from build123d import *

# Parameters (mm, degrees)
CYLINDER010_R     = 2.1
CYLINDER010_DEPTH = 30
CYLINDER011_R     = 2.1
CYLINDER011_DEPTH = 30
SKETCH002_R       = 1.8
SKETCH002_R_2     = 2.1
EXTRUDE001_DEPTH  = 5
BOX010_W          = 7
BOX010_H          = 3.6
BOX010_DEPTH      = 16
FILLET006_R       = 1.5
BOX009_W          = 7
BOX009_H          = 10
BOX009_DEPTH      = 24
FILLET005_R       = 3
SKETCH006_R       = 3
EXTRUDE005_DEPTH  = 9


with BuildPart() as insert_hole:
    # Cylinder010 → Cylinder010 (new body)
    with BuildSketch(Plane(origin=(7.6, 44.5, 0), x_dir=(1, 0, 0), z_dir=(0, 0, 1))):
        Circle(CYLINDER010_R)
    extrude(amount=CYLINDER010_DEPTH)


with BuildPart() as insert_hole_fusion:
    # Cylinder011 → Cylinder011 (new body)
    with BuildSketch(Plane(origin=(9.8, -45.6, 0), x_dir=(1, 0, 0), z_dir=(0, 0, 1))):
        Circle(CYLINDER011_R)
    extrude(amount=CYLINDER011_DEPTH)

    # Fusion010: union insert hole
    add(insert_hole.part)


with BuildPart() as pair_connector_extrude:
    # Sketch002 → Extrude001 (new body)
    with BuildSketch(Plane.XY):
        with BuildLine():
            Line((-36, -49), (0, -49))
            Line((0, -49), (36, -49))
            ThreePointArc((36, -49), (42.363961, -46.363961), (45, -40))
            Line((45, -40), (45, 0))
            Line((45, 0), (45, 40))
            ThreePointArc((45, 40), (42.363961, 46.363961), (36, 49))
            Line((36, 49), (0, 49))
            Line((0, 49), (-36, 49))
            ThreePointArc((-36, 49), (-42.363961, 46.363961), (-45, 40))
            Line((-45, 40), (-45, 0))
            Line((-45, 0), (-45, -40))
            ThreePointArc((-45, -40), (-42.363961, -46.363961), (-36, -49))
        make_face()
        with Locations((-18, 45)):
            Circle(SKETCH002_R, mode=Mode.SUBTRACT)
        with Locations((18, 45)):
            Circle(SKETCH002_R, mode=Mode.SUBTRACT)
        with Locations((-18, -45)):
            Circle(SKETCH002_R, mode=Mode.SUBTRACT)
        with Locations((18, -45)):
            Circle(SKETCH002_R, mode=Mode.SUBTRACT)
        with Locations((-41, 10)):
            Circle(SKETCH002_R_2, mode=Mode.SUBTRACT)
        with Locations((-41, -10)):
            Circle(SKETCH002_R_2, mode=Mode.SUBTRACT)
        with Locations((41, -10)):
            Circle(SKETCH002_R_2, mode=Mode.SUBTRACT)
        with Locations((41, 10)):
            Circle(SKETCH002_R_2, mode=Mode.SUBTRACT)
        with BuildLine():
            Line((-30, -42), (0, -42))
            Line((0, -42), (30, -42))
            ThreePointArc((30, -42), (34.949747, -39.949747), (37, -35))
            Line((37, -35), (37, 0))
            Line((37, 0), (37, 35))
            ThreePointArc((37, 35), (34.949747, 39.949747), (30, 42))
            Line((30, 42), (0, 42))
            Line((0, 42), (-30, 42))
            ThreePointArc((-30, 42), (-34.949747, 39.949747), (-37, 35))
            Line((-37, 35), (-37, 0))
            Line((-37, 0), (-37, -35))
            ThreePointArc((-37, -35), (-34.949747, -39.949747), (-30, -42))
        make_face(mode=Mode.SUBTRACT)
    extrude(amount=EXTRUDE001_DEPTH)


with BuildPart() as pair_connector_extrude_1:
    # Extrude001 placement: moved
    add(pair_connector_extrude.part.moved(Location((0, 0, 6.2))))


with BuildPart() as stand_hole_fillet:
    # Box010 → Box010 (new body)
    with BuildSketch(Plane(origin=(0, -1.8, 4), x_dir=(1, 0, 0), z_dir=(0, 0, 1))):
        with Locations((3.5, 1.8)):
            Rectangle(BOX010_W, BOX010_H)
    extrude(amount=BOX010_DEPTH)

    # Fillet006
    fillet006_edges = [stand_hole_fillet.edges().sort_by_distance(p)[0] for p in [
        (3.5, -1.8, 4),
        (3.5, -1.8, 20),
        (3.5, 1.8, 4),
        (3.5, 1.8, 20),
    ]]
    fillet(fillet006_edges, radius=FILLET006_R)


with BuildPart() as stand_hole_cut:
    # Box009 → Box009 (new body)
    with BuildSketch(Plane(origin=(0, -5, 0), x_dir=(1, 0, 0), z_dir=(0, 0, 1))):
        with Locations((3.5, 5)):
            Rectangle(BOX009_W, BOX009_H)
    extrude(amount=BOX009_DEPTH)

    # Fillet005
    fillet005_edges = [stand_hole_cut.edges().sort_by_distance(p)[0] for p in [
        (3.5, -5, 24),
        (3.5, 5, 24),
    ]]
    fillet(fillet005_edges, radius=FILLET005_R)

    # Cut005: cut stand hole fillet
    add(stand_hole_fillet.part, mode=Mode.SUBTRACT)


with BuildPart() as negative_stand_compound:
    # Compound022 base: copy of stand hole cut
    add(stand_hole_cut.part)


with BuildPart() as negative_stand_compound_1:
    # Compound022 placement: moved
    add(negative_stand_compound.part.moved(Location((-15.1, -45.9, 15.2))))


with BuildPart() as positive_stand_compound:
    # Compound023 base: copy of stand hole cut
    add(stand_hole_cut.part)


with BuildPart() as positive_stand_compound_1:
    # Compound023 placement: moved
    add(positive_stand_compound.part.moved(Location((-8.7, 46, 15.2))))


with BuildPart() as pair_connector_fusion_cut:
    # Sketch006 → Extrude005 (new body)
    with BuildSketch(Plane.XY):
        with BuildLine():
            Line((-22.841771, 51), (23.601032, 51))
            ThreePointArc((25.015246, 49.585786), (24.601032, 50.585786), (23.601032, 51))
            Line((25.015246, 49.585786), (25.015246, 42.214214))
            ThreePointArc((23.801032, 41), (24.659611, 41.355635), (25.015246, 42.214214))
            Line((23.801032, 41), (-23.041771, 41))
            ThreePointArc((-24.255985, 42.214214), (-23.90035, 41.355635), (-23.041771, 41))
            Line((-24.255985, 42.214214), (-24.255985, 49.585786))
            ThreePointArc((-22.841771, 51), (-23.841771, 50.585786), (-24.255985, 49.585786))
        make_face()
        with Locations((18, 45)):
            Circle(SKETCH006_R, mode=Mode.SUBTRACT)
        with Locations((-18, 45)):
            Circle(SKETCH006_R, mode=Mode.SUBTRACT)
        with BuildLine():
            Line((-22.399903, -41), (21.849301, -41))
            ThreePointArc((23.263515, -42.414214), (22.849301, -41.414214), (21.849301, -41))
            Line((23.263515, -42.414214), (23.263515, -49.785786))
            ThreePointArc((22.049301, -51), (22.90788, -50.644365), (23.263515, -49.785786))
            Line((22.049301, -51), (-22.599903, -51))
            ThreePointArc((-23.814117, -49.785786), (-23.458482, -50.644365), (-22.599903, -51))
            Line((-23.814117, -49.785786), (-23.814117, -42.414214))
            ThreePointArc((-22.399903, -41), (-23.399903, -41.414214), (-23.814117, -42.414214))
        make_face()
        with Locations((-18, -45)):
            Circle(SKETCH006_R, mode=Mode.SUBTRACT)
        with Locations((18, -45)):
            Circle(SKETCH006_R, mode=Mode.SUBTRACT)
    extrude(amount=EXTRUDE005_DEPTH)


with BuildPart() as pair_connector_fusion_cut_1:
    # Extrude005 placement: moved
    add(pair_connector_fusion_cut.part.moved(Location((0, 0, 6.2))))

    # Fusion008: union pair connector extrude, negative stand compound, positive stand compound
    add(pair_connector_extrude_1.part)
    add(negative_stand_compound_1.part)
    add(positive_stand_compound_1.part)

    # Cut007: cut insert hole fusion
    add(insert_hole_fusion.part, mode=Mode.SUBTRACT)


solid = pair_connector_fusion_cut_1.part
Read the model definition and answer for the solid it produces. Units are mm, in the model's axes. A direction names the side the tool comes from. Round coordinates to 2 decimals unless told otherwise and drop trailing zeros. Write each loop counter-clockwise with the first axis right and the second up, starting at its lowest first coordinate (ties: lowest second). Pieces come first, ordered by that corner, then holes.
1. Given pin 1 Ø3 at (y, z) = (-48, 33) entering from -X; pin 2 Ø3.5 at (x, y) = (41, -10) entering from +Z; pin 3 Ø10.5 at (x, y) = (-35.5, -5.5) entering from +Z; pin 4 Ø7.5 at (x, z) = (-12.5, 26) entering from -Y, each flat-ended and moving along its own axis, determine where each tip first touches the part or whether it passes through.
2. The part is cut by section C-C, the plane y = -30. Determine the outline of the cut face in (x, z).
3. Straight lines are drawn through the part: L1, parallel to Y at x = 18, z = 14; L2, parallel to X at y = 44.5, z = 10.5; L3, parallel to Y at x = -18, z = 7.6. For each, find the intervals that lie inside material, in ascending order.
4. The part is cut by section D-D, the plane y = 10. Determine the outline of the cut face in (x, z).
5. The part is cut by section A-A, the plane z = 27. Determine the outline of the cut face in (x, y), then the cut area to 3 significant figures.
6. The part is cut by section B-B, the plane x = -18. Determine the outline of the cut face in (y, z).
7. Determine the mould class of faces 1 (the face through (-11.55, -50.04, 38.3)), 2 (the face through (-12, -47.7, 27)), 3 (the face through (-34.9, 40, 8.7)) for opening direction Z: pulls with the +Z half, pulls with the -Z half, needs draft (parallel to the pull), parting line crosses it, or undercut.
8. Which of the six approach directions +Z, -Z, +X, -X, +Y, -Y give full straight-line access (tool end or side, diameter ignored) to faces 4 (the face through (-35, -39.9, 8.7)), 5 (the face through (-18, 48, 13)), 6 (the face through (-12, -44.1, 27)), 7 (the face through (-8.7, 48, 27))?
Values:
1. pin 1: stops at x = -15.1
1. pin 2: passes through
1. pin 3: stops at z = 11.2
1. pin 4: stops at y = -50.9
2. outline: (-45, 6.2) - (-37, 6.2) - (-37, 11.2) - (-45, 11.2) - close; (37, 6.2) - (45, 6.2) - (45, 11.2) - (37, 11.2) - close
3. L1: y = -51 to -48, -42 to -41, 41 to 42, 48 to 51
3. L2: x = -43.79 to -19.73, -16.27 to 5.5, 9.7 to 16.27, 19.73 to 43.79
3. L3: y = -51 to -46.8, -43.2 to -41, 41 to 43.2, 46.8 to 51
4. outline: (-45, 6.2) - (-43.1, 6.2) - (-43.1, 11.2) - (-45, 11.2) - close; (-38.9, 6.2) - (-37, 6.2) - (-37, 11.2) - (-38.9, 11.2) - close; (37, 6.2) - (38.9, 6.2) - (38.9, 11.2) - (37, 11.2) - close; (43.1, 6.2) - (45, 6.2) - (45, 11.2) - (43.1, 11.2) - close
5. outline: (-15.1, -50.9) - (-8.1, -50.9) - (-8.1, -47.7) - (-15.1, -47.7) - close; (-15.1, -44.1) - (-8.1, -44.1) - (-8.1, -40.9) - (-15.1, -40.9) - close; (-8.7, 41) - (-1.7, 41) - (-1.7, 44.2) - (-8.7, 44.2) - close; (-8.7, 47.8) - (-1.7, 47.8) - (-1.7, 51) - (-8.7, 51) - close
5. area: 89.6 mm2
6. outline: (-51, 6.2) - (-46.8, 6.2) - (-46.8, 11.2) - (-48, 11.2) - (-48, 15.2) - (-51, 15.2) - close; (-43.2, 6.2) - (-41, 6.2) - (-41, 15.2) - (-42, 15.2) - (-42, 11.2) - (-43.2, 11.2) - close; (41, 6.2) - (43.2, 6.2) - (43.2, 11.2) - (42, 11.2) - (42, 15.2) - (41, 15.2) - close; (46.8, 6.2) - (51, 6.2) - (51, 15.2) - (48, 15.2) - (48, 11.2) - (46.8, 11.2) - close
7. face 1: pulls with the +Z half
7. face 2: undercut
7. face 3: needs draft
8. face 4: +Z, -Z
8. face 5: +Z
8. face 6: +X, -X
8. face 7: +Z, -X, +Y
